```python
from build123d import *

# Parameters (mm, degrees)
SKETCH1_W                 = 26
SKETCH1_H                 = 71
BOSS_EXTRUDE1_DEPTH       = 6
CUT_EXTRUDE9_REACH        = 40.279
SKETCH10_R                = 2.15
SKETCH11_R                = 3.4
CUT_EXTRUDE10_DEPTH       = 4.2
SKETCH5_R                 = 0.95
CUT_EXTRUDE4_DEPTH        = 5
LPATTERN1_COUNT           = 7
LPATTERN1_PITCH           = 5
LPATTERN2_COPY_1_SKETCH_R = 0.95
LPATTERN2_COPY_1_DEPTH    = 5
LPATTERN2_COPY_2_SKETCH_R = 0.95
LPATTERN2_COPY_2_DEPTH    = 5
LPATTERN2_COPY_3_SKETCH_R = 0.95
LPATTERN2_COPY_3_DEPTH    = 5
LPATTERN2_COPY_4_SKETCH_R = 0.95
LPATTERN2_COPY_4_DEPTH    = 5
LPATTERN2_COPY_5_SKETCH_R = 0.95
LPATTERN2_COPY_5_DEPTH    = 5
LPATTERN2_COPY_6_SKETCH_R = 0.95
LPATTERN2_COPY_6_DEPTH    = 5
LPATTERN2_COPY_7_SKETCH_R = 0.95
LPATTERN2_COPY_7_DEPTH    = 5
LPATTERN2_COPY_8_SKETCH_R = 0.95
LPATTERN2_COPY_8_DEPTH    = 5
FILLET1_R                 = 1


with BuildPart() as part:
    # Sketch1 → Boss-Extrude1 (new body)
    with BuildSketch(Plane(origin=(0, 0, 0), x_dir=(1, 0, 0), z_dir=(0, 1, 0))):
        Rectangle(SKETCH1_W, SKETCH1_H)
    extrude(amount=BOSS_EXTRUDE1_DEPTH)

    # Sketch10 → Cut-Extrude9 (cut, up to next)
    with BuildSketch(Plane(origin=(0, 6, 0), x_dir=(1, 0, 0), z_dir=(0, 1, 0)), mode=Mode.PRIVATE) as cut_extrude9_sk1:
        with Locations(Location((0, -10.5, 0), (0, 0, 270))):
            Circle(SKETCH10_R)
    cut_extrude9_tool1 = extrude(cut_extrude9_sk1.sketch, amount=-CUT_EXTRUDE9_REACH, mode=Mode.PRIVATE) & part.part
    # Sketch10 → Cut-Extrude9 (cut, up to next)
    with BuildSketch(Plane(origin=(0, 6, 0), x_dir=(1, 0, 0), z_dir=(0, 1, 0)), mode=Mode.PRIVATE) as cut_extrude9_sk2:
        with Locations(Location((0, -16, 0), (0, 0, 270))):
            Circle(SKETCH10_R)
    cut_extrude9_tool2 = extrude(cut_extrude9_sk2.sketch, amount=-CUT_EXTRUDE9_REACH, mode=Mode.PRIVATE) & part.part
    # Sketch10 → Cut-Extrude9 (cut, up to next)
    with BuildSketch(Plane(origin=(0, 6, 0), x_dir=(1, 0, 0), z_dir=(0, 1, 0)), mode=Mode.PRIVATE) as cut_extrude9_sk3:
        with Locations(Location((-6.3, -5, 0), (0, 0, 270))):
            Circle(SKETCH10_R)
    cut_extrude9_tool3 = extrude(cut_extrude9_sk3.sketch, amount=-CUT_EXTRUDE9_REACH, mode=Mode.PRIVATE) & part.part
    # Sketch10 → Cut-Extrude9 (cut, up to next)
    with BuildSketch(Plane(origin=(0, 6, 0), x_dir=(1, 0, 0), z_dir=(0, 1, 0)), mode=Mode.PRIVATE) as cut_extrude9_sk4:
        with Locations(Location((6.3, -5, 0), (0, 0, 270))):
            Circle(SKETCH10_R)
    cut_extrude9_tool4 = extrude(cut_extrude9_sk4.sketch, amount=-CUT_EXTRUDE9_REACH, mode=Mode.PRIVATE) & part.part
    add(cut_extrude9_tool1.solids().sort_by_distance((0, 6, 10.5))[0], mode=Mode.SUBTRACT)
    add(cut_extrude9_tool2.solids().sort_by_distance((0, 6, 16))[0], mode=Mode.SUBTRACT)
    add(cut_extrude9_tool3.solids().sort_by_distance((-6.3, 6, 5))[0], mode=Mode.SUBTRACT)
    add(cut_extrude9_tool4.solids().sort_by_distance((6.3, 6, 5))[0], mode=Mode.SUBTRACT)

    # Sketch11 → Cut-Extrude10 (cut)
    with BuildSketch(Plane(origin=(0, 6, 0), x_dir=(1, 0, 0), z_dir=(0, 1, 0))):
        with Locations(Location((-6.3, -5, 0), (0, 0, 270))):
            Circle(SKETCH11_R)
        with Locations(Location((6.3, -5, 0), (0, 0, 270))):
            Circle(SKETCH11_R)
        with BuildLine():
            Line((3.4, -10.5), (3.4, -16))
            ThreePointArc((3.4, -16), (0, -19.4), (-3.4, -16))
            Line((-3.4, -16), (-3.4, -10.5))
            ThreePointArc((-3.4, -10.5), (0, -7.1), (3.4, -10.5))
        make_face()
    extrude(amount=-CUT_EXTRUDE10_DEPTH, mode=Mode.SUBTRACT)

    # Sketch5 → Cut-Extrude4 (cut)
    with BuildSketch(Plane(origin=(0, 6, 0), x_dir=(1, 0, 0), z_dir=(0, 1, 0))):
        with Locations(Location((-10, 32.5, 0), (0, 0, 270))):
            Circle(SKETCH5_R)
        with Locations(Location((10, 32.5, 0), (0, 0, 270))):
            Circle(SKETCH5_R)
    cut_extrude4 = extrude(amount=-CUT_EXTRUDE4_DEPTH, mode=Mode.SUBTRACT)

    # LPattern1: Cut-Extrude4 ×7
    with Locations(*[(0, 0, i * LPATTERN1_PITCH) for i in range(1, LPATTERN1_COUNT)]):
        add(cut_extrude4, mode=Mode.SUBTRACT)

    # Mirror2: Cut-Extrude4 across plane
    add(cut_extrude4.mirror(Plane.XY), mode=Mode.SUBTRACT)

    # LPattern2 copy 1 sketch → LPattern2 copy 1 (cut)
    with BuildSketch(Plane(origin=(0, 6, -5), x_dir=(1, 0, 0), z_dir=(0, 1, 0))):
        with Locations((-10, -32.5)):
            Circle(LPATTERN2_COPY_1_SKETCH_R)
        with Locations((10, -32.5)):
            Circle(LPATTERN2_COPY_1_SKETCH_R)
    extrude(amount=-LPATTERN2_COPY_1_DEPTH, mode=Mode.SUBTRACT)

    # LPattern2 copy 2 sketch → LPattern2 copy 2 (cut)
    with BuildSketch(Plane(origin=(0, 6, -10), x_dir=(1, 0, 0), z_dir=(0, 1, 0))):
        with Locations((-10, -32.5)):
            Circle(LPATTERN2_COPY_2_SKETCH_R)
        with Locations((10, -32.5)):
            Circle(LPATTERN2_COPY_2_SKETCH_R)
    extrude(amount=-LPATTERN2_COPY_2_DEPTH, mode=Mode.SUBTRACT)

    # LPattern2 copy 3 sketch → LPattern2 copy 3 (cut)
    with BuildSketch(Plane(origin=(0, 6, -15), x_dir=(1, 0, 0), z_dir=(0, 1, 0))):
        with Locations((-10, -32.5)):
            Circle(LPATTERN2_COPY_3_SKETCH_R)
        with Locations((10, -32.5)):
            Circle(LPATTERN2_COPY_3_SKETCH_R)
    extrude(amount=-LPATTERN2_COPY_3_DEPTH, mode=Mode.SUBTRACT)

    # LPattern2 copy 4 sketch → LPattern2 copy 4 (cut)
    with BuildSketch(Plane(origin=(0, 6, -20), x_dir=(1, 0, 0), z_dir=(0, 1, 0))):
        with Locations((-10, -32.5)):
            Circle(LPATTERN2_COPY_4_SKETCH_R)
        with Locations((10, -32.5)):
            Circle(LPATTERN2_COPY_4_SKETCH_R)
    extrude(amount=-LPATTERN2_COPY_4_DEPTH, mode=Mode.SUBTRACT)

    # LPattern2 copy 5 sketch → LPattern2 copy 5 (cut)
    with BuildSketch(Plane(origin=(0, 6, -5), x_dir=(1, 0, 0), z_dir=(0, 1, 0))):
        with Locations(Location((-10, 32.5, 0), (0, 0, 270))):
            Circle(LPATTERN2_COPY_5_SKETCH_R)
        with Locations(Location((10, 32.5, 0), (0, 0, 270))):
            Circle(LPATTERN2_COPY_5_SKETCH_R)
    extrude(amount=-LPATTERN2_COPY_5_DEPTH, mode=Mode.SUBTRACT)

    # LPattern2 copy 6 sketch → LPattern2 copy 6 (cut)
    with BuildSketch(Plane(origin=(0, 6, -10), x_dir=(1, 0, 0), z_dir=(0, 1, 0))):
        with Locations(Location((-10, 32.5, 0), (0, 0, 270))):
            Circle(LPATTERN2_COPY_6_SKETCH_R)
        with Locations(Location((10, 32.5, 0), (0, 0, 270))):
            Circle(LPATTERN2_COPY_6_SKETCH_R)
    extrude(amount=-LPATTERN2_COPY_6_DEPTH, mode=Mode.SUBTRACT)

    # LPattern2 copy 7 sketch → LPattern2 copy 7 (cut)
    with BuildSketch(Plane(origin=(0, 6, -15), x_dir=(1, 0, 0), z_dir=(0, 1, 0))):
        with Locations(Location((-10, 32.5, 0), (0, 0, 270))):
            Circle(LPATTERN2_COPY_7_SKETCH_R)
        with Locations(Location((10, 32.5, 0), (0, 0, 270))):
            Circle(LPATTERN2_COPY_7_SKETCH_R)
    extrude(amount=-LPATTERN2_COPY_7_DEPTH, mode=Mode.SUBTRACT)

    # LPattern2 copy 8 sketch → LPattern2 copy 8 (cut)
    with BuildSketch(Plane(origin=(0, 6, -20), x_dir=(1, 0, 0), z_dir=(0, 1, 0))):
        with Locations(Location((-10, 32.5, 0), (0, 0, 270))):
            Circle(LPATTERN2_COPY_8_SKETCH_R)
        with Locations(Location((10, 32.5, 0), (0, 0, 270))):
            Circle(LPATTERN2_COPY_8_SKETCH_R)
    extrude(amount=-LPATTERN2_COPY_8_DEPTH, mode=Mode.SUBTRACT)

    # Fillet1
    fillet1_edges = [part.edges().sort_by_distance(p)[0] for p in [
        (13, 3, 35.5),
        (-13, 3, 35.5),
        (-13, 3, -35.5),
        (13, 3, -35.5),
    ]]
    fillet(fillet1_edges, radius=FILLET1_R)


solid = part.part
```
Work out the finished part from the listing and answer in its coordinate system (mm). A direction names the side the tool comes from. Give positions to 0.01 mm unless a question says otherwise; leave off trailing zeros. Write each loop counter-clockwise with the first axis right and the second up, starting at its lowest first coordinate (ties: lowest second). Pieces come first, ordered by that corner, then holes.
(1) Straight lines are drawn through the part: line 1 (X direction, y = 3.5, z = -32.5); line 2 (X direction, y = 4.1, z = 15); line 3 (X direction, y = 4.2, z = 23). For each, find the intervals that lie inside material, in ascending order.
Final values:
line 1: x = -13 to -10.95, -9.05 to 9.05, 10.95 to 13
line 2: x = -13 to -3.4, 3.4 to 13
line 3: x = -13 to -10.81, -9.19 to 9.19, 10.81 to 13
(2) Which of the six approach directions +Z, -Z, +X, -X, +Y, -Y give full straight-line access (tool end or side, diameter ignored) to faces 4 (the cylindrical face through (7.753, 0.913, 3.415)), 5 (the cylindrical face through (-9.96, 3.54, -8.45))?
Final values:
face 4: +Y, -Y
face 5: +Y
(3) The mould has two halves that part along Z. Classify faces 1 (the cylindrical face through (10.942, 3.535, -12.624)), 2 (the flat face through (0, 6, 0)), 3 (the flat face through (-10, 1, -28)): pulls with the +Z half, pulls with the -Z half, needs draft (parallel to the pull), parting line crosses it, or undercut.
Final values:
face 1: undercut
face 2: needs draft
face 3: undercut
(4) The part is cut by section B-B on z = 32.5. Write down the section's boundary in (x, y).
Final values:
outline: (-13, 0) - (13, 0) - (13, 6) - (10.95, 6) - (10.95, 1) - (9.05, 1) - (9.05, 6) - (-9.05, 6) - (-9.05, 1) - (-10.95, 1) - (-10.95, 6) - (-13, 6) - close
(5) The part is cut by section A-A on x = -7.25. Write down the section's boundary in (y, z).
Final values:
outline: (0, -35.5) - (6, -35.5) - (6, 1.74) - (1.8, 1.74) - (1.8, 3.07) - (0, 3.07) - close; (0, 6.93) - (1.8, 6.93) - (1.8, 8.26) - (6, 8.26) - (6, 35.5) - (0, 35.5) - close
(6) The part is cut by section C-C on y = 3.7. Count the separate pieces of the cut face and the enclosed holes in it, plus the area to 3 significant figures.
Final values:
separate pieces: 1
enclosed holes: 27
area: 1,630 mm2
(7) Flat-ended cylindrical pins translate along their axes: pin 1 Ø0.6 at (x, z) = (-10, 27.5) entering from +Y; pin 2 Ø2 at (x, z) = (7, 6) entering from +Y. Find the tip coordinate at first contact, or state that the pin passes through.
Final values:
pin 1: stops at y = 1
pin 2: stops at y = 1.8
